Input: part model. Units: mm. Frame: model coordinates. A direction names the side the tool comes from. Round coordinates to 2 decimals unless told otherwise and drop trailing zeros.
1) Draft query along X for faces 4 (the face through (2, -4.45, 8)), 5 (the face through (2.58, 0.35, -2.51)). Return one class per face: pulls with the +X half, pulls with the -X half, needs draft (parallel to the pull), parting line crosses it, or undercut.
2) Ray query, line 1 along Z through (x, y) = (0, 0.95); line 2 along Z through (x, y) = (-0.5, 1.25); line 3 along X through (y, z) = (0.5, -1.25). Return the intervals inside material, ascending.
3) First-contact query: pin 1 (3 mm diameter, centred on x = -1.77, z = -1.77, fed in from +Y); pin 2 (1.3 mm diameter, centred on x = -1.77, z = 1.77, fed in from +Y); pin 3 (3 mm diameter, centred on x = -9.5, y = -0.5, fed in from -Z); pin 4 (2 mm diameter, centred on x = 4.75, z = 0, fed in from -Y). Flat tips, straight axial feed; report the tip coordinate or a pass-through.
4) Access query for faces 1 (the face through (5.55, 0.65, -0.04)), 2 (the face through (9, 1.5, -4)), 3 (the face through (6.512, -2.581, -2.7)). Directions: +Z, -Z, +X, -X, +Y, -Y. A direction counts if a zero-diameter tool reaches every point of the face in a straight line with its end or side. Return the directions, or none.
from build123d import *

# Parameters (mm, degrees)
SKETCH1_R                                       = 12.5
BOSS_EXTRUDE1_DEPTH                             = 1.5
SKETCH2_R                                       = 0.75
CUT_EXTRUDE1_DEPTH                              = 1
CUT_EXTRUDE1_DEPTH_BACK                         = 2.5
CSK_FOR_M2_FLAT_HEAD_MACHINE_SCREW1_D           = 2.2
CSK_FOR_M2_FLAT_HEAD_MACHINE_SCREW1_DEPTH       = 5
CSK_FOR_M2_FLAT_HEAD_MACHINE_SCREW1_CSINK_D     = 3.8
CSK_FOR_M2_FLAT_HEAD_MACHINE_SCREW1_CSINK_ANGLE = 90
CSK_FOR_M2_FLAT_HEAD_MACHINE_SCREW1_TIP         = 0.660946681
SKETCH7_R                                       = 12.5
SKETCH7_R_2                                     = 7.05
BOSS_EXTRUDE2_DEPTH                             = 3.3
SKETCH15_R                                      = 8.5
SKETCH15_R_2                                    = 7.3
BOSS_EXTRUDE4_DEPTH                             = 2
FILLET1_R                                       = 1
CHAMFER1_SIZE                                   = 0.5
CHAMFER2_SIZE                                   = 1
CHAMFER3_SIZE                                   = 2
CHAMFER3_SIZE2                                  = 3.464101615
M2X0_4_TAPPED_HOLE1_D                           = 1.6
M2X0_4_TAPPED_HOLE1_DEPTH                       = 5.2
M2X0_4_TAPPED_HOLE1_CSINK_D                     = 2.05
M2X0_4_TAPPED_HOLE1_CSINK_ANGLE                 = 90
M2X0_4_TAPPED_HOLE1_TIP                         = 0.480688495
CHAMFER4_SIZE                                   = 0.8


with BuildPart() as part:
    # Sketch1 → Boss-Extrude1 (new body)
    with BuildSketch(Plane(origin=(0, 0, 0), x_dir=(1, 0, 0), z_dir=(0, 1, 0))):
        Circle(SKETCH1_R)
    extrude(amount=BOSS_EXTRUDE1_DEPTH)

    # Sketch2 → Cut-Extrude1 (cut, two sides)
    with BuildSketch(Plane(origin=(0, 1.5, 0), x_dir=(1, 0, 0), z_dir=(0, 1, 0))) as cut_extrude1_sk:
        Circle(SKETCH2_R)
    extrude(amount=CUT_EXTRUDE1_DEPTH, mode=Mode.SUBTRACT)
    extrude(cut_extrude1_sk.sketch, amount=-CUT_EXTRUDE1_DEPTH_BACK, mode=Mode.SUBTRACT)

    # CSK for M2 Flat Head Machine Screw1
    with Locations(Plane(origin=(0, 1.5, 0), x_dir=(1, 0, 0), z_dir=(0, 1, 0))):
        with Locations((-1.767766953, 1.767766953), (1.767766953, 1.767766953), (1.767766953, -1.767766953), (-1.767766953, -1.767766953)):
            CounterSinkHole(CSK_FOR_M2_FLAT_HEAD_MACHINE_SCREW1_D / 2, CSK_FOR_M2_FLAT_HEAD_MACHINE_SCREW1_CSINK_D / 2, depth=CSK_FOR_M2_FLAT_HEAD_MACHINE_SCREW1_DEPTH, counter_sink_angle=CSK_FOR_M2_FLAT_HEAD_MACHINE_SCREW1_CSINK_ANGLE)
            with Locations((0, 0, -(CSK_FOR_M2_FLAT_HEAD_MACHINE_SCREW1_DEPTH + CSK_FOR_M2_FLAT_HEAD_MACHINE_SCREW1_TIP / 2))):  # 118° drill point
                Cone(0, CSK_FOR_M2_FLAT_HEAD_MACHINE_SCREW1_D / 2, CSK_FOR_M2_FLAT_HEAD_MACHINE_SCREW1_TIP, mode=Mode.SUBTRACT)

    # Sketch6 → Revolve1 (revolve)
    with BuildSketch(Plane.XY):
        Polygon((-12.5, 0), (-12.5, -1.15), (-7.05, -1.15), (-5, 0), align=None)
    revolve(axis=Axis((0, 0, 0), (0, -1, 0)))

    # Sketch7 → Boss-Extrude2 (add)
    with BuildSketch(Plane.XZ.offset(1.15)):
        Circle(SKETCH7_R)
        Circle(SKETCH7_R_2, mode=Mode.SUBTRACT)
    extrude(amount=BOSS_EXTRUDE2_DEPTH)

    # Sketch15 → Boss-Extrude4 (add)
    with BuildSketch(Plane(origin=(0, 1.5, 0), x_dir=(1, 0, 0), z_dir=(0, 1, 0))):
        Circle(SKETCH15_R)
        Circle(SKETCH15_R_2, mode=Mode.SUBTRACT)
    extrude(amount=BOSS_EXTRUDE4_DEPTH)

    # Fillet1
    fillet1_edges = [part.edges().sort_by_distance(p)[0] for p in [
        (0, -1.15, 7.05),
        (5, 0, 0),
        (-7.3, 1.5, 0),
        (-8.5, 1.5, 0),
    ]]
    fillet(fillet1_edges, radius=FILLET1_R)

    # Chamfer1
    chamfer1_edges = [part.edges().sort_by_distance(p)[0] for p in [
        (-12.5, 1.5, 0),
    ]]
    chamfer(chamfer1_edges, length=CHAMFER1_SIZE)

    # Chamfer2
    chamfer2_edges = [part.edges().sort_by_distance(p)[0] for p in [
        (-7.05, -4.45, 0),
    ]]
    chamfer(chamfer2_edges, length=CHAMFER2_SIZE)

    # Chamfer3
    chamfer3_edges = [part.edges().sort_by_distance(p)[0] for p in [
        (-12.5, -4.45, 0),
    ]]
    chamfer3_side = [part.faces().sort_by_distance(p)[0] for p in [
        (-8.403553391, -4.45, 0),
    ]]
    chamfer(chamfer3_edges, length=CHAMFER3_SIZE, length2=CHAMFER3_SIZE2, reference=chamfer3_side[0])

    # M2x0.4 Tapped Hole1
    with Locations(Plane(origin=(0, 1.5, 0), x_dir=(1, 0, 0), z_dir=(0, 1, 0))):
        with Locations((-4.75, 0), (4.75, 0)):
            CounterSinkHole(M2X0_4_TAPPED_HOLE1_D / 2, M2X0_4_TAPPED_HOLE1_CSINK_D / 2, depth=M2X0_4_TAPPED_HOLE1_DEPTH, counter_sink_angle=M2X0_4_TAPPED_HOLE1_CSINK_ANGLE)
            with Locations((0, 0, -(M2X0_4_TAPPED_HOLE1_DEPTH + M2X0_4_TAPPED_HOLE1_TIP / 2))):  # 118° drill point
                Cone(0, M2X0_4_TAPPED_HOLE1_D / 2, M2X0_4_TAPPED_HOLE1_TIP, mode=Mode.SUBTRACT)

    # Chamfer4
    chamfer4_edges = [part.edges().sort_by_distance(p)[0] for p in [
        (-8.5, 3.5, 0),
    ]]
    chamfer(chamfer4_edges, length=CHAMFER4_SIZE)


solid = part.part
Final values:
1. face 4: needs draft
1. face 5: undercut
2. line 1: z = -12.5 to -0.75, 0.75 to 12.5
2. line 2: z = -12.24 to -2.82, -0.71 to -0.56, 0.56 to 0.71, 2.82 to 12.24
2. line 3: x = -12.44 to -2.74, -0.8 to 0.8, 2.74 to 12.44
3. pin 1: stops at y = 1.1
3. pin 2: passes through
3. pin 3: stops at z = -9.6
3. pin 4: stops at y = -0.42
4. face 1: +Y, -Y
4. face 2: +Y
4. face 3: -Y
